```python
from build123d import *

# Parameters (mm, degrees)
F0_W     = 35
F0_H     = 50
F1_DEPTH = 10.25
F2_W     = 21
F2_H     = 19
F3_DEPTH = 25
F5_W     = 50.25
F5_H     = 74
F6_DEPTH = 5.08


with BuildPart() as f1:
    # F0 (on Front) → F1 (new body)
    with BuildSketch(Plane.XZ):
        Rectangle(F0_W, F0_H)
    extrude(amount=F1_DEPTH)

    # F2 (on face) → F3 (cut)
    with BuildSketch(Plane.XZ.offset(10.25)):
        with Locations((0, 15.5)):
            Rectangle(F2_W, F2_H)
    extrude(amount=-F3_DEPTH, mode=Mode.SUBTRACT)

    # F5 (on offset) → F6 (join)
    with BuildSketch(Plane(origin=(0, 0, -25), x_dir=(1, 0, 0), z_dir=(0, 0, -1))):
        with Locations((0, 16.5)):
            Rectangle(F5_W, F5_H)
    extrude(amount=F6_DEPTH)


solid = f1.part
```
Part model, mm, in its own coordinate system. A direction names the side the tool comes from. Round coordinates to 2 decimals unless told otherwise and drop trailing zeros. Order: outer loops, then holes, each group sorted by start corner. A loop starts at its lowest first (then second) coordinate and runs counter-clockwise, first axis right, second up. Notation, with made-up numbers: M 31.25,0.25 L 78.25,0.25 A31 ccw 78.25,26.25 Z; hole C -7,-24 d1. An arc over 180 degrees is marked long. Answer in a Markdown table with one row per item. Add a question column.
Q1. Cut at B-B on x = 16. Give the cut face in (y, z), and give its area (3 significant figures).
Q2. 3-axis set-ups, long thin cutter, end or side, ignore diameter. For faces 4 (the face through (-17.5, -5, 0)), 5 (the face through (0, -10.25, -5)), 6 (the face through (0, 0, -5)), 7 (the face through (10.5, -5, 15)): which of +Z, -Z, +X, -X, +Y, -Y reach the whole face in a straight line?
Q3. Cut at C-C on y = 15. Give the cut face in (x, z) (3 decimals).
Q4. Pin check, flat tips, straight feed: pin 1 (5 mm diameter, centred on y = -4.5, z = 16.5, fed in from +X); pin 2 (8 mm diameter, centred on y = -2.5, z = 6, fed in from -X); pin 3 (17.5 mm diameter, centred on x = 8.5, z = -2.5, fed in from -Y); pin 4 (4 mm diameter, centred on y = -35, z = -21.5, fed in from +X). Stop position of each tip, or through.
Q5. Wall check: L1, parallel to X at y = -4.5, z = 18.5; L2, parallel to Z at x = 19.5, y = -44; L3, parallel to Y at x = 16.5, z = 6. Give the ranges that are in metal, low to high. Write a range as from..to.
Q6. Mould opens along X. For faces 1 (the face through (0, -17, -30.08)), 2 (the face through (17.5, -5, 0)), 3 (the face through (0, -5, 6)) say: +X half, -X half, draft (parallel to the pull), parting line (faces both ways), or undercut.
Q7. Cut at A-A on z = 20. Give the cut face in (x, y), and give its area (4 significant figures).
Q8. Cut at D-D on x = 3.5. Give the cut face in (y, z), and give its area (3 significant figures).
Established:
| question | item | result |
|---|---|---|
| 1 | outline | M -53.5,-30.08 L 20.5,-30.08 L 20.5,-25 L 0,-25 L 0,25 L -10.25,25 L -10.25,-25 L -53.5,-25 Z |
| 1 | area | 888 mm2 |
| 2 | face 4 | +Z, -X, +Y, -Y |
| 2 | face 5 | +Z, +X, -X, -Y |
| 2 | face 6 | +Z, +X, -X, +Y |
| 2 | face 7 | +Z, +Y, -Y |
| 3 | outline | M -25.125,-30.08 L 25.125,-30.08 L 25.125,-25 L -25.125,-25 Z |
| 4 | pin 1 | stops at x = 17.5 |
| 4 | pin 2 | stops at x = -17.5 |
| 4 | pin 3 | stops at y = -10.25 |
| 4 | pin 4 | passes through |
| 5 | L1 | x = -17.5..-10.5, 10.5..17.5 |
| 5 | L2 | z = -30.08..-25 |
| 5 | L3 | y = -10.25..0 |
| 6 | face 1 | draft |
| 6 | face 2 | +X half |
| 6 | face 3 | undercut |
| 7 | outline | M -17.5,-10.25 L -10.5,-10.25 L -10.5,0 L -17.5,0 Z; M 10.5,-10.25 L 17.5,-10.25 L 17.5,0 L 10.5,0 Z |
| 7 | area | 143.5 mm2 |
| 8 | outline | M -53.5,-30.08 L 20.5,-30.08 L 20.5,-25 L 0,-25 L 0,6 L -10.25,6 L -10.25,-25 L -53.5,-25 Z |
| 8 | area | 694 mm2 |
